The model under review builds one solid part; all positions refer to its coordinate system, in mm. Face numbers are marked on the shaded views. Coordinates: 2 decimals unless noted, no trailing zeros. Write each loop counter-clockwise with the first axis right and the second up, starting at its lowest first coordinate (ties: lowest second). Pieces come first, ordered by that corner, then holes. Notation, with made-up numbers: M -4.75,-18.75 L 46.25,-18.75 A33 cw 46.25,14.25 Z; hole C 84,77 d10. An arc over 180 degrees is marked long. Answer as a JSON object with one key per item and string values.
```python
from build123d import *

# Parameters (mm, degrees)
SKETCH1_W           = 42.7
SKETCH1_H           = 22.51
BOSS_EXTRUDE1_DEPTH = 11.37
FILLET1_R           = 2.5
SKETCH2_R           = 1.26
SKETCH2_R_2         = 2.32
CUT_EXTRUDE1_DEPTH  = 12


with BuildPart() as part:
    # Sketch1 → Boss-Extrude1 (new body)
    with BuildSketch(Plane.XY):
        Rectangle(SKETCH1_W, SKETCH1_H)
    extrude(amount=BOSS_EXTRUDE1_DEPTH)

    # Fillet1
    fillet1_edges = [part.edges().sort_by_distance(p)[0] for p in [
        (0, -11.255, 11.37),
        (0, -11.255, 0),
        (0, 11.255, 0),
        (0, 11.255, 11.37),
    ]]
    fillet(fillet1_edges, radius=FILLET1_R)

    # Sketch2 → Cut-Extrude1 (cut)
    with BuildSketch(Plane(origin=(21.35, 0, 0), x_dir=(0, 0, -1), z_dir=(1, 0, 0))):
        with Locations((-5.784105099, 5.852044752)):
            Circle(SKETCH2_R)
        with Locations((-5.784105099, -2.931681994)):
            Circle(SKETCH2_R_2)
    extrude(amount=-CUT_EXTRUDE1_DEPTH, mode=Mode.SUBTRACT)


solid = part.part
```
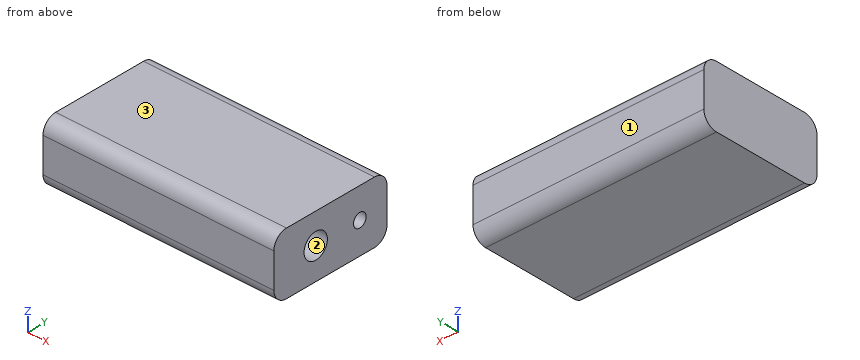
(1) Wall thickness on line 1 along Y through (x, z) = (15, 5.25) (3 decimals); line 2 along Z through (x, y) = (16, -4); line 3 along Z through (x, y) = (-17, 9.25): over which ranges is each line inside the solid? List them lowest first. Write a range as from..to.
Results list:
{"line 1": "-11.255..-5.189, -0.674..4.711, 6.993..11.255", "line 2": "0..3.72, 7.84..11.37", "line 3": "0.05..11.32"}
(2) Add section C-C on y = -4. Give the boundary of the cut face in (x, z).
Results list:
{"outline": "M -21.35,0 L 21.35,0 L 21.35,3.72 L 9.35,3.72 L 9.35,7.84 L 21.35,7.84 L 21.35,11.37 L -21.35,11.37 Z"}
(3) Add section B-B on z = 6.5. Give the boundary of the cut face in (x, y) (3 decimals).
Results list:
{"outline": "M -21.35,-11.255 L 21.35,-11.255 L 21.35,-5.138 L 9.35,-5.138 L 9.35,-0.725 L 21.35,-0.725 L 21.35,4.815 L 9.35,4.815 L 9.35,6.889 L 21.35,6.889 L 21.35,11.255 L -21.35,11.255 Z"}
(4) For pin 1 Ø2.5 at (y, z) = (-3, 5.5) entering from +X, flat-tipped, find the tip position at first contact; note if it passes through.
Results list:
{"pin 1": "x = 9.35"}
(5) Add section D-D on x = 15.5. Give the boundary of the cut face in (y, z) (3 decimals).
Results list:
{"outline": "M -11.255,2.5 A2.5 ccw -8.755,0 L 8.755,0 A2.5 ccw 11.255,2.5 L 11.255,8.87 A2.5 ccw 8.755,11.37 L -8.755,11.37 A2.5 ccw -11.255,8.87 Z; hole C -2.932,5.784 d4.64; hole C 5.852,5.784 d2.52"}
(6) Add section A-A on x = 2. Give the boundary of the cut face in (y, z) (3 decimals), and give its area (3 significant figures).
Results list:
{"outline": "M -11.255,2.5 A2.5 ccw -8.755,0 L 8.755,0 A2.5 ccw 11.255,2.5 L 11.255,8.87 A2.5 ccw 8.755,11.37 L -8.755,11.37 A2.5 ccw -11.255,8.87 Z", "area": "251 mm²"}
(7) Draft analysis for pull direction Y (two halves, no side actions). For the marked faces 1, 2 and 3, state which applies: released by +Y, released by -Y, zero draft, split by the parting line, or undercut.
Results list:
{"face 1": "released by +Y", "face 2": "undercut", "face 3": "zero draft"}
